Geometry check sheet. Reference: drawing and pictorial views, mm from the part's lowest x, y, z. Give positions to 0.01 mm unless a question says otherwise; leave off trailing zeros. Loops run counter-clockwise (first coordinate to the right, second up) from the corner with the lowest first, then second, coordinate; pieces in that order, holes last. Notation, with made-up numbers: (16, 47.25) -> (69, 47.25) arc R24 cw to (69, 82.25) -> close; hole circle Ø10 at (-8, -39). An arc over 180 degrees is marked (long way). One line per item, written item: value. Start each with the question number.
(1) Sectioned sample at B-B, the plane z = 107.5. Record the cut outline in (x, y), then the cut area to 3 significant figures.
(2) Sectioned sample at A-A, the plane x = 4.5. Record the cut outline in (y, z).
(3) Gauge pin test, flat ends, axial feed: pin 1 Ø0.6 at (y, z) = (1.5, 121) entering from -X; pin 2 Ø0.6 at (x, y) = (63, 1) entering from +Z; pin 3 Ø0.6 at (y, z) = (1, 2) entering from +X; pin 4 Ø2 at (x, z) = (49, 81) entering from -Y. Record the tip position at first contact, or that the pin passes through.
(4) Scan lines: line 1 along X through (y, z) = (1.3, 38); line 2 along Z through (x, y) = (40, 0.95). Record each from-to range of solid material in increasing order. Write a range as from..to.
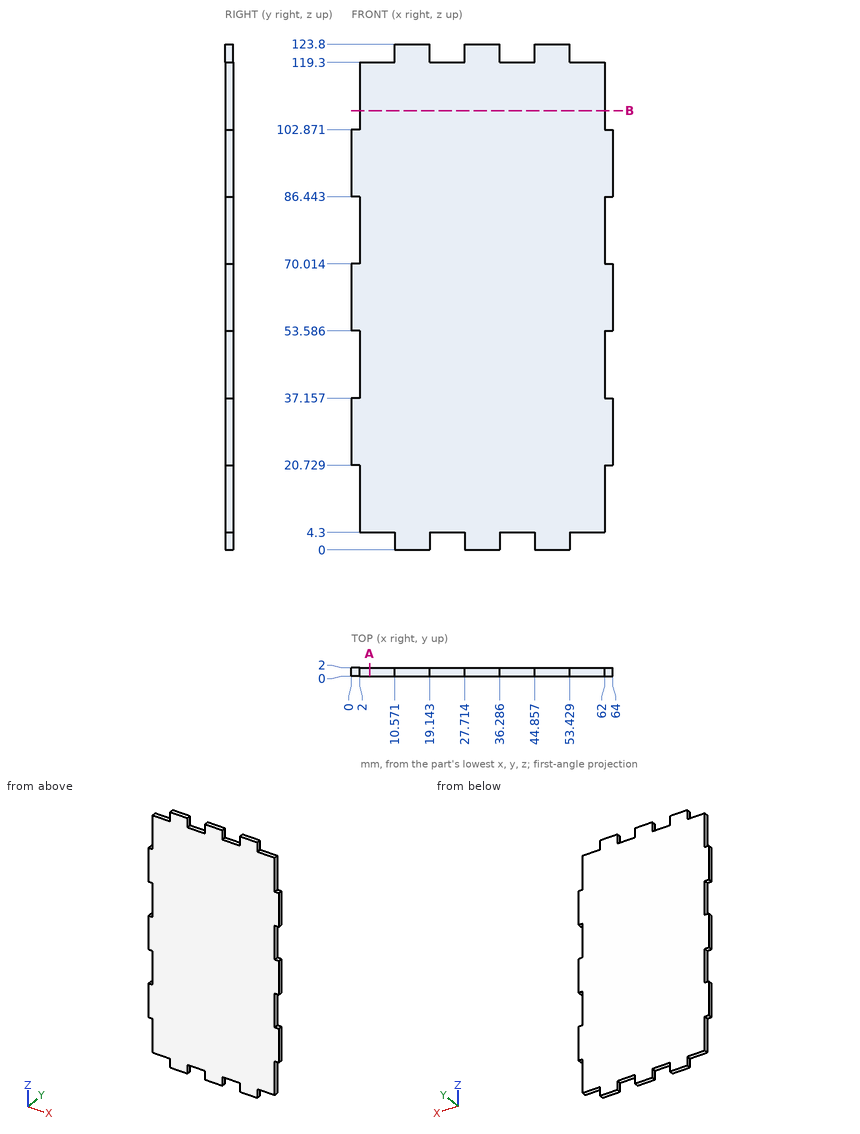
Calculated:
1. outline: (2, 0) -> (62, 0) -> (62, 2) -> (2, 2) -> close
1. area: 120 mm2
2. outline: (0, 4.3) -> (2, 4.3) -> (2, 119.3) -> (0, 119.3) -> close
3. pin 1: stops at x = 10.57
3. pin 2: stops at z = 102.87
3. pin 3: stops at x = 53.43
3. pin 4: stops at y = 0
4. line 1: x = 2..62
4. line 2: z = 4.3..119.3
